Source: CAD feature listing. Evaluate the final solid. Frame: model axes, mm. Face numbers are marked on the shaded views. A direction names the side the tool comes from. Coordinates: 2 decimals unless noted, no trailing zeros. Write item = value, one per line. Start each with the question number.
Item 1: Mould query, pull axis Y, two halves, no side actions, for the marked faces 3, 4 and 5. Classes: released by +Y, released by -Y, zero draft, split by the parting line, or undercut.
Item 2: Contact query for flat-ended pins moving along their axis: pin 1 (5.5 mm diameter, centred on x = 22, z = 1.5, fed in from +Y); pin 2 (4 mm diameter, centred on x = 10, z = 17, fed in from +Y); pin 3 (1 mm diameter, centred on x = 18, y = 11.5, fed in from +Z). Output: stop coordinate, or through.
Item 3: Set-up query: the marked faces 1 and 2. Return all of +Z, -Z, +X, -X, +Y, -Y with unobstructed straight access to the full face (end or side cutting, diameter ignored); none if empty.
Item 4: Section query A-A (y = 7.5). Count the separate pieces of the cut face and the enclosed holes in it, then the cut area to 3 significant figures.
Item 5: Ray query, line 1 along X through (y, z) = (7.5, 10); line 2 along Y through (x, z) = (32.5, 10.75); line 3 along X through (y, z) = (6.5, 3.75). Return the intervals inside material, ascending. Write a range as [from, to].
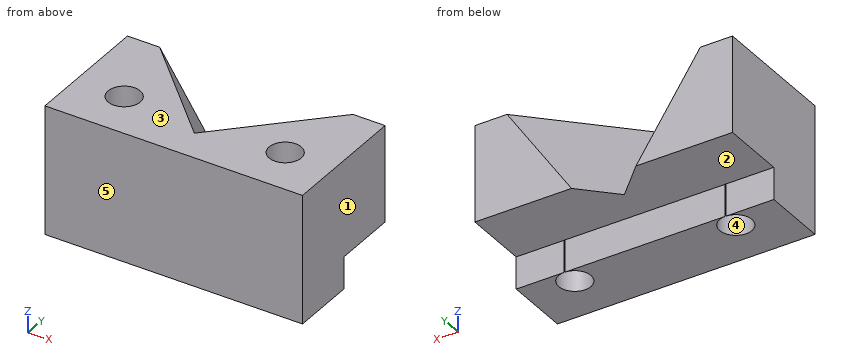
```python
from build123d import *

# Parameters (mm, degrees)
IZIM1_W                     = 40
IZIM1_H                     = 20
Y_KSEKLIK_EKSTR_ZYON1_DEPTH = 20
IZIM2_R                     = 2.5
KES_EKSTR_ZYON1_DEPTH       = 20
IZIM3_W                     = 40
IZIM3_H                     = 5
KES_EKSTR_ZYON3_DEPTH       = 9
IZIM6_W                     = 40
IZIM6_H                     = 5
KES_EKSTR_ZYON13_DEPTH      = 1.001


with BuildPart() as part:
    # Çizim1 → Yükseklik-Ekstrüzyon1 (new body)
    with BuildSketch(Plane.XY):
        with Locations((20, 10)):
            Rectangle(IZIM1_W, IZIM1_H)
    extrude(amount=Y_KSEKLIK_EKSTR_ZYON1_DEPTH)

    # Çizim2 → Kes-Ekstrüzyon1 (cut)
    with BuildSketch(Plane.XY.offset(20)):
        with Locations((7.5, 7.5)):
            Circle(IZIM2_R)
        with Locations((32.5, 7.5)):
            Circle(IZIM2_R)
    extrude(amount=-KES_EKSTR_ZYON1_DEPTH, mode=Mode.SUBTRACT)

    # Çizim3 → Kes-Ekstrüzyon3 (cut)
    with BuildSketch(Plane(origin=(0, 20, 0), x_dir=(1, 0, 0), z_dir=(0, 1, 0))):
        with Locations((20, -2.5)):
            Rectangle(IZIM3_W, IZIM3_H)
    extrude(amount=-KES_EKSTR_ZYON3_DEPTH, mode=Mode.SUBTRACT)

    # Çizim5 → Kes-Loft2 section 0
    with BuildSketch(Plane(origin=(0, 0, 5), x_dir=(-1, 0, 0), z_dir=(0, 0, -1))):
        Polygon((-25, 20), (-20, 15), (-15, 20), align=None)
    # Çizim4 → Kes-Loft2 section 1
    with BuildSketch(Plane.XY.offset(20)):
        Polygon((5, 20), (20, 5), (35, 20), align=None)
    loft(mode=Mode.SUBTRACT)

    # Çizim6 → Kes-Ekstrüzyon13 (cut)
    with BuildSketch(Plane(origin=(0, 11, 0), x_dir=(1, 0, 0), z_dir=(0, 1, 0))):
        with Locations((20, -2.5)):
            Rectangle(IZIM6_W, IZIM6_H)
    extrude(amount=-KES_EKSTR_ZYON13_DEPTH, mode=Mode.SUBTRACT)


solid = part.part
```
Computed:
q1.face_3 = zero draft
q1.face_4 = undercut
q1.face_5 = released by -Y
q2.pin_1 = 10
q2.pin_2 = 19.4
q2.pin_3 = 14.31
q3.face_1 = +Z, -Z, +X, +Y, -Y
q3.face_2 = -Z, +X, -X, +Y
q4.separate_pieces = 3
q4.enclosed_holes = 0
q4.area = 591 mm^2
q5.line_1 = [0, 5], [10, 30], [35, 40]
q5.line_2 = [0, 5], [10, 20]
q5.line_3 = [0, 5.21], [9.79, 30.21], [34.79, 40]
